Source: three-view drawing plus pictorial views. Frame: mm from the lowest corner of the part. Round coordinates to 2 decimals unless told otherwise and drop trailing zeros. Loops run counter-clockwise (first coordinate to the right, second up) from the corner with the lowest first, then second, coordinate; pieces in that order, holes last. Notation, with made-up numbers: M -14,8.5 L 31,8.5 A26 ccw 31,34.5 Z; hole C -30,-8 d6. An arc over 180 degrees is marked long. Answer as a JSON object with one key per item and string values.
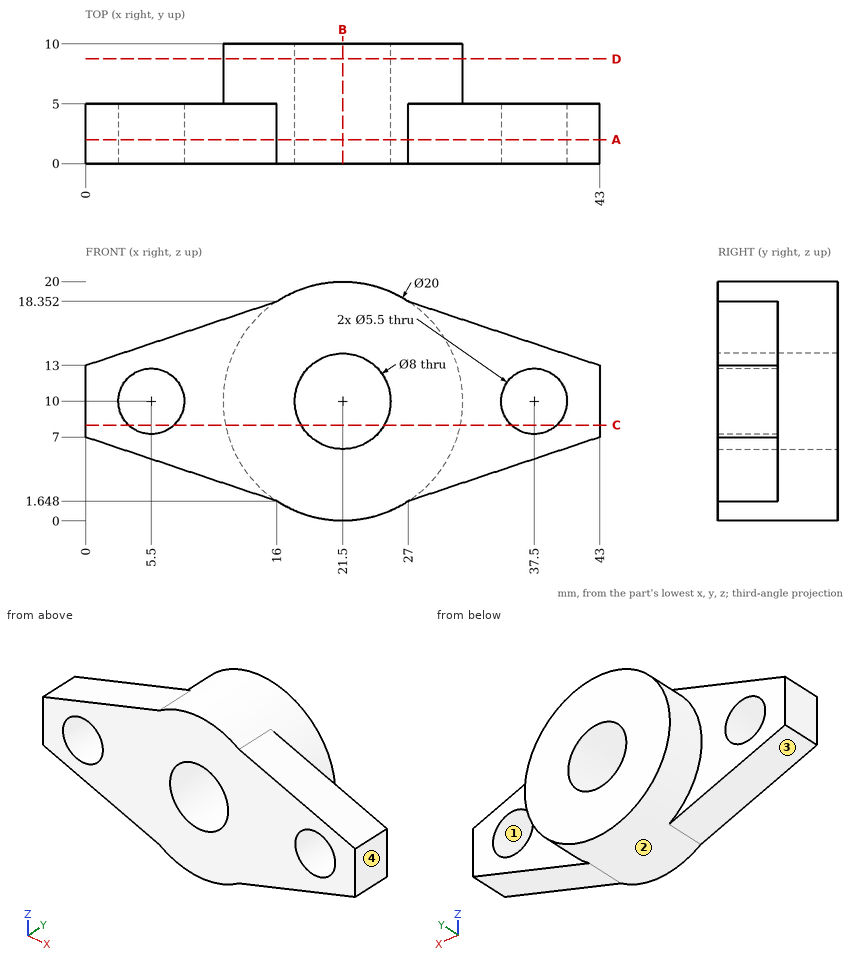
1) Cut plane C-C on z = 8. Return the cut outline in (x, y).
Geometry results:
{"outline": "M 0,0 L 3.61,0 L 3.61,5 L 0,5 Z; M 7.39,0 L 18.04,0 L 18.04,10 L 11.7,10 L 11.7,5 L 7.39,5 Z; M 24.96,0 L 35.61,0 L 35.61,5 L 31.3,5 L 31.3,10 L 24.96,10 Z; M 39.39,0 L 43,0 L 43,5 L 39.39,5 Z"}
2) First-contact query: pin 1 (9 mm diameter, centred on x = 5.5, z = 10, fed in from -Y); pin 2 (7 mm diameter, centred on x = 21.5, z = 10, fed in from +Y); pin 3 (3 mm diameter, centred on x = 7, z = 13, fed in from +Y); pin 4 (1 mm diameter, centred on x = 6.5, y = 3.5, fed in from +Z). Flat tips, straight axial feed; report the tip coordinate or a pass-through.
Geometry results:
{"pin 1": "y = 0", "pin 2": "through", "pin 3": "y = 5", "pin 4": "z = 15.34"}
3) Cut plane D-D on y = 8.75. Return the cut outline in (x, z).
Geometry results:
{"outline": "C 21.5,10 d20; hole C 21.5,10 d8"}
4) Cut plane B-B on x = 21.5. Return the cut outline in (y, z), and give its area (3 significant figures).
Geometry results:
{"outline": "M 0,0 L 10,0 L 10,6 L 0,6 Z; M 0,14 L 10,14 L 10,20 L 0,20 Z", "area": "120 mm2"}
5) Cut plane A-A on y = 2. Return the cut outline in (x, z).
Geometry results:
{"outline": "M 0,7 L 16,1.65 A10 ccw 27,1.65 L 43,7 L 43,13 L 27,18.35 A10 ccw 16,18.35 L 0,13 Z; hole C 5.5,10 d5.5; hole C 21.5,10 d8; hole C 37.5,10 d5.5"}
6) Pull-direction query (X, two-part tool) for the marked faces 1, 2, 3 and 4; classes: +X half, -X half, draft (parallel to the pull), parting line (faces both ways), or undercut.
Geometry results:
{"face 1": "undercut", "face 2": "parting line", "face 3": "-X half", "face 4": "+X half"}
7) Line query: probe 1 along X at (y, z) = (1.3, 10); probe 2 along X at (y, z) = (7, 10); probe 3 along Y at (x, z) = (12.5, 16.75). Output: solid intervals per line, ascending.
Geometry results:
{"probe 1": "0 to 2.75, 8.25 to 17.5, 25.5 to 34.75, 40.25 to 43", "probe 2": "11.5 to 17.5, 25.5 to 31.5", "probe 3": "0 to 5"}
